The model under review builds one solid part; all positions refer to its coordinate system, in mm. A direction names the side the tool comes from. Coordinates: 2 decimals unless noted, no trailing zeros. Write each loop counter-clockwise with the first axis right and the second up, starting at its lowest first coordinate (ties: lowest second). Pieces come first, ordered by that corner, then holes.
1) Add section A-A, the plane z = 10. State the section outline as (x, y) points, then the cut area to 3 significant figures.
2) Mouldability with a two-part tool opening along X and no side actions: class faces 4 (the flat face through (67.3, 1.5, 11.8)), 5 (the flat face through (63, 1, 20)), 6 (the flat face through (60.159, 1, 0)) as released by +X, released by -X, zero draft, split by the parting line, or undercut.
3) Add section D-D, the plane x = 68. State the section outline as (y, z) points.
4) Machinability: for faces 1 (the flat face through (65, 1, -15)), 2 (the flat face through (65, 1, 15)), 3 (the flat face through (69.8, 1, 0)), which of the approach directions +Z, -Z, +X, -X, +Y, -Y give a long, thin tool a straight path to every point of the face, cutting with its end or side? Answer none if there is none.
5) For P1, Ø1.5, axis at x = 66.5, z = -14.5, coming from the +Y side, flat-tipped, find the tip position at first contact; note if it passes through.
6) Add section B-B, the plane y = 2.25. State the section outline as (x, z) points.
7) Add section C-C, the plane z = -11. State the section outline as (x, y) points, then the cut area to 3 significant figures.
8) For line 1 (X direction, y = 2.2, z = 14); line 2 (Z direction, x = 67.25, y = 0.95); line 3 (X direction, y = 2.5, z = -15), list the stretches that pass through material, from the lowest coordinate up.
from build123d import *

# Parameters (mm, degrees)
CROQUIS1_R                 = 11
CROQUIS1_R_2               = 2
CROQUIS1_W                 = 30
CROQUIS1_H                 = 3
SALIENTE_EXTRUIR1_DEPTH    = 3
CROQUIS2_R                 = 13
CROQUIS2_R_2               = 11
SALIENTE_EXTRUIR2_DEPTH    = 4
CROQUIS3_R                 = 13
CROQUIS3_R_2               = 9
SALIENTE_EXTRUIR3_DEPTH    = 2
CHAFL_N1_SIZE              = 2
CHAFL_N2_SIZE              = 10
CORTAR_EXTRUIR1_DEPTH      = 10
CORTAR_EXTRUIR1_DEPTH_BACK = 10
CROQUIS4_W                 = 128.833311542
CROQUIS4_H                 = 58.233807115
REDONDEO1_R                = 0.1


with BuildPart() as part:
    # Croquis1 → Saliente-Extruir1 (new body)
    with BuildSketch(Plane(origin=(0, 0, 0), x_dir=(1, 0, 0), z_dir=(0, 1, 0))):
        Polygon((65, 9.5), (69.8, 14.3), (69.8, -14.3), (65, -9.5), (65, -20), (-65, -20), (-65, 20), (65, 20), align=None)
        with Locations(Location((-50.129942902, 0, 0), (0, 0, 270))):
            Circle(CROQUIS1_R, mode=Mode.SUBTRACT)
        with Locations(Location((-28.595127909, 0, 0), (0, 0, 270))):
            Circle(CROQUIS1_R_2, mode=Mode.SUBTRACT)
        with Locations(Location((-13.595127909, 0, 0), (0, 0, 270))):
            Circle(CROQUIS1_R_2, mode=Mode.SUBTRACT)
        with Locations(Location((50, 0, 0), (0, 0, 270))):
            Circle(CROQUIS1_R_2, mode=Mode.SUBTRACT)
        with Locations((25, 11)):
            Rectangle(CROQUIS1_W, CROQUIS1_H, mode=Mode.SUBTRACT)
        with Locations((25, -11)):
            Rectangle(CROQUIS1_W, CROQUIS1_H, mode=Mode.SUBTRACT)
    extrude(amount=SALIENTE_EXTRUIR1_DEPTH)

    # Croquis2 → Saliente-Extruir2 (add)
    with BuildSketch(Plane(origin=(0, 3, 0), x_dir=(1, 0, 0), z_dir=(0, 1, 0))):
        with Locations(Location((-50.129942902, 0, 0), (0, 0, 90))):
            Circle(CROQUIS2_R)
        with Locations(Location((-50.129942902, 0, 0), (0, 0, 270))):
            Circle(CROQUIS2_R_2, mode=Mode.SUBTRACT)
    extrude(amount=SALIENTE_EXTRUIR2_DEPTH)

    # Croquis3 → Saliente-Extruir3 (add)
    with BuildSketch(Plane(origin=(0, 7, 0), x_dir=(1, 0, 0), z_dir=(0, 1, 0))):
        with Locations(Location((-50.129942902, 0, 0), (0, 0, 90))):
            Circle(CROQUIS3_R)
        with Locations(Location((-50.129942902, 0, 0), (0, 0, 270))):
            Circle(CROQUIS3_R_2, mode=Mode.SUBTRACT)
    extrude(amount=SALIENTE_EXTRUIR3_DEPTH)

    # Chafl_n1
    chafl_n1_edges = [part.edges().sort_by_distance(p)[0] for p in [
        (-50.129942902, 9, 13),
    ]]
    chamfer(chafl_n1_edges, length=CHAFL_N1_SIZE)

    # Chafl_n2
    chafl_n2_edges = [part.edges().sort_by_distance(p)[0] for p in [
        (-65, 1.5, 20),
        (-65, 1.5, -20),
    ]]
    chamfer(chafl_n2_edges, length=CHAFL_N2_SIZE)

    # Croquis4 → Cortar-Extruir1 (cut, two sides: drawn at the far end of the back side and taken through both)
    with BuildSketch(Plane(origin=(0, 3, 0), x_dir=(1, 0, 0), z_dir=(0, 1, 0)).offset(-CORTAR_EXTRUIR1_DEPTH_BACK)):
        with Locations((-4.257997369, -0.71893589)):
            Rectangle(CROQUIS4_W, CROQUIS4_H)
    extrude(amount=CORTAR_EXTRUIR1_DEPTH + CORTAR_EXTRUIR1_DEPTH_BACK, mode=Mode.SUBTRACT)

    # Redondeo1
    redondeo1_edges = [part.edges().sort_by_distance(p)[0] for p in [
        (69.8, 1.5, -14.3),
        (69.8, 1.5, 14.3),
    ]]
    fillet(redondeo1_edges, radius=REDONDEO1_R)


solid = part.part
Geometry results:
1. outline: (60.16, 0) - (65, 0) - (65, 3) - (60.16, 3) - close; (65.5, 0) - (69.8, 0) - (69.8, 3) - (65.5, 3) - close
1. area: 27.4 mm2
2. face 4: undercut
2. face 5: zero draft
2. face 6: released by -X
3. outline: (0, -12.5) - (3, -12.5) - (3, 12.5) - (0, 12.5) - close
4. face 1: -Z, +Y, -Y
4. face 2: +Z, +Y, -Y
4. face 3: +Z, -Z, +X, +Y, -Y
5. P1: passes through
6. outline: (60.16, -20) - (65, -20) - (65, -9.5) - (69.63, -14.13) arc R0.1 ccw to (69.8, -14.06) - (69.8, 14.06) arc R0.1 ccw to (69.63, 14.13) - (65, 9.5) - (65, 20) - (60.16, 20) - close
7. outline: (60.16, 0) - (65, 0) - (65, 3) - (60.16, 3) - close; (66.5, 0) - (69.8, 0) - (69.8, 3) - (66.5, 3) - close
7. area: 24.4 mm2
8. line 1: x = 60.16 to 65, 69.5 to 69.8
8. line 2: z = -11.75 to 11.75
8. line 3: x = 60.16 to 65
